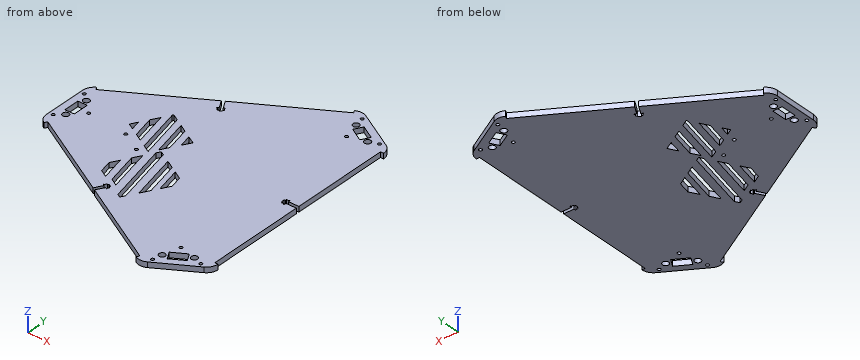
```python
from build123d import *

# Parameters (mm, degrees)
SKETCH1_R           = 3
SKETCH1_R_2         = 1.5
SKETCH1_W           = 9
SKETCH1_H           = 15
BOSS_EXTRUDE1_DEPTH = 5
CUT_EXTRUDE1_DEPTH  = 6
CUT_EXTRUDE2_DEPTH  = 6
CUT_EXTRUDE3_DEPTH  = 10
SKETCH4_R           = 1.5
CUT_EXTRUDE4_DEPTH  = 10


with BuildPart() as part:
    # Sketch1 → Boss-Extrude1 (new body)
    with BuildSketch(Plane.XY):
        with BuildLine():
            Line((-127.0125, 27.949853865), (39.300966521, 123.970978531))
            Line((39.300966521, 123.970978531), (37.800966521, 126.569054742))
            ThreePointArc((37.800966521, 126.569054742), (43.313466521, 128.046124665), (48.825966521, 126.569054742))
            Line((48.825966521, 126.569054742), (85.199033479, 105.569054742))
            ThreePointArc((85.199033479, 105.569054742), (89.234463556, 101.533624665), (90.711533479, 96.021124665))
            Line((90.711533479, 96.021124665), (87.711533479, 96.021124665))
            Line((87.711533479, 96.021124665), (87.711533479, -96.021124665))
            Line((87.711533479, -96.021124665), (90.711533479, -96.021124665))
            ThreePointArc((90.711533479, -96.021124665), (89.234463556, -101.533624665), (85.199033479, -105.569054742))
            Line((85.199033479, -105.569054742), (48.825966521, -126.569054742))
            ThreePointArc((48.825966521, -126.569054742), (43.313465898, -128.046124665), (37.800965443, -126.56905412))
            Line((37.800965443, -126.56905412), (39.300965736, -123.970978078))
            Line((39.300965736, -123.970978078), (-127.012489947, -27.949834641))
            Line((-127.012489947, -27.949834641), (-128.512501078, -30.547929455))
            ThreePointArc((-128.512501078, -30.547929455), (-132.547930388, -26.512499461), (-134.025, -21))
            Line((-134.025, -21), (-134.025, 21))
            ThreePointArc((-134.025, 21), (-132.547930077, 26.5125), (-128.5125, 30.547930077))
            Line((-128.5125, 30.547930077), (-127.0125, 27.949853865))
        make_face()
        with Locations((-123, 12)):
            Circle(SKETCH1_R, mode=Mode.SUBTRACT)
        with Locations((-123, -12)):
            Circle(SKETCH1_R, mode=Mode.SUBTRACT)
        with Locations((71.892304845, 100.521124665)):
            Circle(SKETCH1_R, mode=Mode.SUBTRACT)
        with Locations((51.107695155, 112.521124665)):
            Circle(SKETCH1_R, mode=Mode.SUBTRACT)
        with Locations((51.107695155, -112.521124665)):
            Circle(SKETCH1_R, mode=Mode.SUBTRACT)
        with Locations((71.892304845, -100.521124665)):
            Circle(SKETCH1_R, mode=Mode.SUBTRACT)
        with Locations((-111, 0)):
            Circle(SKETCH1_R_2, mode=Mode.SUBTRACT)
        with Locations((55.5, 96.12881982)):
            Circle(SKETCH1_R_2, mode=Mode.SUBTRACT)
        with Locations((55.5, -96.12881982)):
            Circle(SKETCH1_R_2, mode=Mode.SUBTRACT)
        with Locations((-130, 18)):
            Circle(SKETCH1_R_2, mode=Mode.SUBTRACT)
        with Locations((-130, -18)):
            Circle(SKETCH1_R_2, mode=Mode.SUBTRACT)
        with Locations((80.588457268, 103.583302492)):
            Circle(SKETCH1_R_2, mode=Mode.SUBTRACT)
        with Locations((49.411542732, 121.583302492)):
            Circle(SKETCH1_R_2, mode=Mode.SUBTRACT)
        with Locations((49.411542732, -121.583302492)):
            Circle(SKETCH1_R_2, mode=Mode.SUBTRACT)
        with Locations((80.588457268, -103.583302492)):
            Circle(SKETCH1_R_2, mode=Mode.SUBTRACT)
        Polygon((57.254809472, -114.168238983), (70.245190528, -106.668238983), (65.745190528, -98.874010348), (52.754809472, -106.374010348), align=None, mode=Mode.SUBTRACT)
        with Locations((-123, 0)):
            Rectangle(SKETCH1_W, SKETCH1_H, mode=Mode.SUBTRACT)
        Polygon((65.745190528, 98.874010348), (52.754809472, 106.374010348), (57.254809472, 114.168238983), (70.245190528, 106.668238983), align=None, mode=Mode.SUBTRACT)
    extrude(amount=BOSS_EXTRUDE1_DEPTH)

    # Sketch2 → Cut-Extrude1 (cut, through all)
    with BuildSketch(Plane.XY.offset(5)):
        Polygon((87.711533479, 1.48), (77.711533479, 1.48), (77.711533479, 3.5), (77.211533479, 3.5), (77.211533479, 2.75), (74.711533479, 2.75), (74.711533479, 1.48), (73.711533479, 1.48), (73.711533479, -1.48), (74.711533479, -1.48), (74.711533479, -2.75), (77.211533479, -2.75), (77.211533479, -3.5), (77.711533479, -3.5), (77.711533479, -1.48), (87.711533479, -1.48), align=None)
        Polygon((-43.223568195, -77.825416198), (-38.223568195, -69.16516216), (-36.474196879, -70.17516216), (-36.224196879, -69.742149458), (-36.873715932, -69.367149458), (-35.623715932, -67.202085949), (-36.723568195, -66.567085949), (-36.223568195, -65.701060545), (-38.78700339, -64.221060545), (-39.28700339, -65.087085949), (-40.386855653, -64.452085949), (-41.636855653, -66.617149458), (-42.286374706, -66.242149458), (-42.536374706, -66.67516216), (-40.78700339, -67.68516216), (-45.78700339, -76.345416198), align=None)
        Polygon((-46.436522443, 75.220416198), (-41.436522443, 66.56016216), (-43.185893759, 65.55016216), (-42.935893759, 65.117149458), (-42.286374706, 65.492149458), (-41.036374706, 63.327085949), (-39.936522443, 63.962085949), (-39.436522443, 63.096060545), (-36.873087248, 64.576060545), (-37.373087248, 65.442085949), (-36.273234985, 66.077085949), (-37.523234985, 68.242149458), (-36.873715932, 68.617149458), (-37.123715932, 69.05016216), (-38.873087248, 68.04016216), (-43.873087248, 76.700416198), align=None)
    extrude(amount=-CUT_EXTRUDE1_DEPTH, mode=Mode.SUBTRACT)

    # Sketch3 → Cut-Extrude2 (cut, through all)
    with BuildSketch(Plane.XY.offset(5)):
        Polygon((-57.539549529, -41.661428389), (-54.909843958, -53.412518972), (-47.84919289, -57.488988829), (-53.108604032, -33.986807663), align=None)
        Polygon((-48.677658535, -26.312186937), (-41.678771487, -57.587382375), (-34.618120419, -61.663852232), (-44.246713038, -18.637566211), align=None)
        Polygon((-39.093651522, -9.712204179), (-25.516557684, -70.382745138), (-22.133329048, -72.336053611), (-19.825544935, -68.338855316), (-33.293067707, -8.157943131), (-36.970490138, -6.034781747), align=None)
        Polygon((-25.081734637, -12.898759725), (-14.672483419, -59.413493284), (-9.856238314, -51.071514234), (-17.407113911, -17.329705222), align=None)
        Polygon((-11.868595954, -20.527370889), (-6.380514763, -45.05138602), (-1.564269657, -36.70940697), (-4.193975228, -24.958316386), align=None)
    extrude(amount=-CUT_EXTRUDE2_DEPTH, mode=Mode.SUBTRACT)

    # Sketch5 → Cut-Extrude3 (cut)
    with BuildSketch(Plane.XY.offset(5)):
        Polygon((-40.061292463, -5.388208187), (-48.069042542, 30.395188095), (-41.008391474, 26.318718238), (-35.630346966, 2.286412538), align=None)
        Polygon((-66.256008164, 29.241209516), (-58.864982983, -3.786292638), (-65.92563405, 0.290177219), (-70.686953661, 21.56658879), align=None)
        Polygon((-33.947740407, 22.242248381), (-31.199401469, 9.961033264), (-26.568563639, 17.981877577), align=None)
        Polygon((-55.12969361, 34.471657952), (-44.743680847, -11.939232352), (-51.804331915, -7.862762495), (-61.825062667, 36.915830242), (-61.209577533, 37.981881487), align=None)
        Polygon((-75.117899158, 13.891968064), (-72.986285118, 4.366647077), (-78.709580954, 7.670994329), align=None)
    extrude(amount=-CUT_EXTRUDE3_DEPTH, mode=Mode.SUBTRACT)

    # Sketch4 → Cut-Extrude4 (cut)
    with BuildSketch(Plane.XY.offset(5)):
        with Locations((-72.175794174, -4.380771204)):
            Circle(SKETCH4_R)
        with Locations((-53.162424939, -15.35814505)):
            Circle(SKETCH4_R)
    extrude(amount=-CUT_EXTRUDE4_DEPTH, mode=Mode.SUBTRACT)


solid = part.part
```
Could you check a few things on this model? Use its own coordinates, in mm. Give positions to 0.01 mm unless a question says otherwise; leave off trailing zeros. Loops run counter-clockwise (first coordinate to the right, second up) from the corner with the lowest first, then second, coordinate; pieces in that order, holes last. Notation, with made-up numbers: (2.5, 74.25) -> (54.5, 74.25) arc R22 ccw to (54.5, 108.25) -> close; hole circle Ø2 at (-13, -28.5). An arc over 180 degrees is marked (long way). Put each result on its own line as item: value.
(1) Imagine slicing it at B-B on z = 2. State how many separate pieces and enclosed holes the cut face has, plus the area to 3 significant figures.
Computed:
separate pieces: 1
enclosed holes: 30
area: 34,500 mm^2
(2) Imagine slicing it at A-A on x = -123. Write out the boundary of the cut face in (y, z).
Computed:
outline: (-30.27, 0) -> (-15, 0) -> (-15, 5) -> (-30.27, 5) -> close; (-9, 0) -> (-7.5, 0) -> (-7.5, 5) -> (-9, 5) -> close; (7.5, 0) -> (9, 0) -> (9, 5) -> (7.5, 5) -> close; (15, 0) -> (30.27, 0) -> (30.27, 5) -> (15, 5) -> close
(3) I'm going to push flat-ended pins straight in: pin 1 Ø2.5 at (x, y) = (80.59, 103.58) entering from +Z; pin 2 Ø1.5 at (x, z) = (45, 3) entering from -Y; pin 3 Ø0.5 at (x, z) = (74.5, 2.5) entering from +Y; pin 4 Ø0.6 at (y, z) = (-2, 3) entering from +X. Where does each tip first touch, or does it pass through?
Computed:
pin 1: through
pin 2: y = -128.01
pin 3: y = 111.89
pin 4: x = 87.71
(4) Please list where these lines run through material, in increasing order: probe 1 along X at (y, z) = (-54, 1.45); probe 2 along Y at (x, z) = (-123, 3); probe 3 along X at (y, z) = (110, 1.05). Write a range as [from, to].
Computed:
probe 1: [-81.89, -53.89], [-48.63, -42.48], [-36.33, -29.18], [-23.03, -15.88], [-11.55, 87.71]
probe 2: [-30.27, -15], [-9, -7.5], [7.5, 9], [15, 30.27]
probe 3: [15.1, 49.48], [52.73, 54.85], [64.47, 77.52]
(5) Imagine slicing it at C-C on x = 9. Write out the boundary of the cut face in (y, z), plus the area to 3 significant figures.
Computed:
outline: (-106.48, 0) -> (106.48, 0) -> (106.48, 5) -> (-106.48, 5) -> close
area: 1,060 mm^2
